from build123d import *

# Parameters (mm, degrees)
F1_DEPTH = 3
F2_DEPTH = 2.5
F3_R     = 4.5
F4_DEPTH = 1.25
F6_SIZE  = 1.24999
F5_R     = 1.75
F7_DEPTH = 1.35


# Not quite as in the source:
# - a fillet or chamfer is up to 0.001 mm smaller than in the source, because OpenCascade refuses the exact size


with BuildPart() as f1:
    # F0 (on Top) → F1 (new body)
    with BuildSketch(Plane.XY):
        with BuildLine():
            ThreePointArc((7.8345588235, -1.6185450382), (6.75, 0), (7.8345588235, 1.6185450382))
            ThreePointArc((7.8345588235, 1.6185450382), (7.7274066103, 2.0705523608), (7.5941994877, 2.5155782915))
            ThreePointArc((7.5941994877, 2.5155782915), (5.8456714755, 3.375), (5.9756544495, 5.318980532))
            ThreePointArc((5.9756544495, 5.318980532), (5.6568542495, 5.6568542495), (5.318980532, 5.9756544495))
            ThreePointArc((5.318980532, 5.9756544495), (3.375, 5.8456714755), (2.5155782915, 7.5941994877))
            ThreePointArc((2.5155782915, 7.5941994877), (2.0705523608, 7.7274066103), (1.6185450382, 7.8345588235))
            ThreePointArc((1.6185450382, 7.8345588235), (0, 6.75), (-1.6185450382, 7.8345588235))
            ThreePointArc((-1.6185450382, 7.8345588235), (-2.0705523608, 7.7274066103), (-2.5155782915, 7.5941994877))
            ThreePointArc((-2.5155782915, 7.5941994877), (-2.5038989162, 7.4779678276), (-2.5, 7.3612159322))
            ThreePointArc((-2.5, 7.3612159322), (-3.4780595655, 5.7906720883), (-5.318980532, 5.9756544495))
            ThreePointArc((-5.318980532, 5.9756544495), (-5.6568542495, 5.6568542495), (-5.9756544495, 5.318980532))
            ThreePointArc((-5.9756544495, 5.318980532), (-5.7048294141, 4.8146978862), (-5.6112159322, 4.25))
            ThreePointArc((-5.6112159322, 4.25), (-6.2090920721, 2.932764026), (-7.5941994877, 2.5155782915))
            ThreePointArc((-7.5941994877, 2.5155782915), (-7.7274066103, 2.0705523608), (-7.8345588235, 1.6185450382))
            ThreePointArc((-7.8345588235, 1.6185450382), (-7.0462080515, 0.9741606493), (-6.75, 0))
            ThreePointArc((-6.75, 0), (-7.0462080515, -0.9741606493), (-7.8345588235, -1.6185450382))
            ThreePointArc((-7.8345588235, -1.6185450382), (-7.7274066103, -2.0705523608), (-7.5941994877, -2.5155782915))
            ThreePointArc((-7.5941994877, -2.5155782915), (-6.2090920721, -2.932764026), (-5.6112159322, -4.25))
            ThreePointArc((-5.6112159322, -4.25), (-5.7048294141, -4.8146978862), (-5.9756544495, -5.318980532))
            ThreePointArc((-5.9756544495, -5.318980532), (-5.6568542495, -5.6568542495), (-5.318980532, -5.9756544495))
            ThreePointArc((-5.318980532, -5.9756544495), (-3.4780595655, -5.7906720883), (-2.5, -7.3612159322))
            ThreePointArc((-2.5, -7.3612159322), (-2.5038989162, -7.4779678276), (-2.5155782915, -7.5941994877))
            ThreePointArc((-2.5155782915, -7.5941994877), (-2.0705523608, -7.7274066103), (-1.6185450382, -7.8345588235))
            ThreePointArc((-1.6185450382, -7.8345588235), (0, -6.75), (1.6185450382, -7.8345588235))
            ThreePointArc((1.6185450382, -7.8345588235), (2.0705523608, -7.7274066103), (2.5155782915, -7.5941994877))
            ThreePointArc((2.5155782915, -7.5941994877), (3.375, -5.8456714755), (5.318980532, -5.9756544495))
            ThreePointArc((5.318980532, -5.9756544495), (5.6568542495, -5.6568542495), (5.9756544495, -5.318980532))
            ThreePointArc((5.9756544495, -5.318980532), (5.8456714755, -3.375), (7.5941994877, -2.5155782915))
            ThreePointArc((7.5941994877, -2.5155782915), (7.7274066103, -2.0705523608), (7.8345588235, -1.6185450382))
        make_face()
        Polygon((3.4641016151, 0), (1.7320508076, -3), (-1.7320508076, -3), (-3.4641016151, 0), (-1.7320508076, 3), (1.7320508076, 3), align=None, mode=Mode.SUBTRACT)
        Polygon((-1.7320508076, -3), (1.7320508076, -3), (3.4641016151, 0), (1.7320508076, 3), (-1.7320508076, 3), (-3.4641016151, 0), align=None)
    extrude(amount=F1_DEPTH)

    # F0 (on Top) → F2 (cut)
    with BuildSketch(Plane.XY):
        Polygon((-1.7320508076, -3), (1.7320508076, -3), (3.4641016151, 0), (1.7320508076, 3), (-1.7320508076, 3), (-3.4641016151, 0), align=None)
    extrude(amount=F2_DEPTH, mode=Mode.SUBTRACT)

    # F3 (on face) → F4 (join)
    with BuildSketch(Plane.XY.offset(3)):
        Circle(F3_R)
    extrude(amount=F4_DEPTH)

    # F6 (size 1.25 in the source; OpenCascade refuses exactly that, so slightly less here)
    f6_edges = [f1.edges().sort_by_distance(p)[0] for p in [
        (-4.5, 0, 4.25),
    ]]
    chamfer(f6_edges, length=F6_SIZE)

    # F5 (on face) → F7 (cut)
    with BuildSketch(Plane.XY.offset(4.25)):
        Circle(F5_R)
    extrude(amount=-F7_DEPTH, mode=Mode.SUBTRACT)


solid = f1.part
Input: part model. Units: mm. Frame: model coordinates. A direction names the side the tool comes from. Round coordinates to 2 decimals unless told otherwise and drop trailing zeros. Write each loop counter-clockwise with the first axis right and the second up, starting at its lowest first coordinate (ties: lowest second). Pieces come first, ordered by that corner, then holes.
1) Reachability of faces 4 (the flat face through (0, 0, 2.9)), 5 (the cylindrical face through (-7.726, 2.077, 1.479)), 6 (the flat face through (-2.6, -1.5, 1.2)) from +Z, -Z, +X, -X, +Y, -Y: full face, straight path, thin tool, end or side. Return the list, or none.
2) Draft query along Y for faces 1 (the cylindrical face through (2.06, -7.73, 1.48)), 2 (the cylindrical face through (1.617, -0.67, 3.584)), 3 (the flat face through (-4, 0, 0)). Return one class per face: pulls with the +Y half, pulls with the -Y half, needs draft (parallel to the pull), parting line crosses it, or undercut.
3) Cut plane B-B (z = 4.05). Return the cut outline in (x, y), then the cut area to 3 significant figures.
4) Contact query for flat-ended pins moving along their axis: P1, Ø1, axis at x = 0.5, y = 0, coming from the +Z side; P2, Ø3, axis at x = 0, y = 0, coming from the -Z side; P3, Ø1.2, axis at x = -0.5, z = 1, coming from the -Y side. Output: stop coordinate, or through.
5) Cut plane C-C (y = 6.25). Return the cut outline in (x, z), then the cut area to 3 significant figures.
6) Ray query, L1, parallel to Z at x = -2, y = 0.25; L2, parallel to Z at x = -7, y = -1; L3, parallel to Y at x = 0, z = 3.95. Return the intervals inside material, ascending.
Geometry says:
1. face 4: +Z
1. face 5: +Z, -Z, -X, +Y
1. face 6: -Z
2. face 1: pulls with the -Y half
2. face 2: undercut
2. face 3: needs draft
3. outline: circle Ø6.9 at (0, 0); hole circle Ø3.5 at (0, 0)
3. area: 27.8 mm2
4. P1: stops at z = 2.9
4. P2: stops at z = 2.5
4. P3: stops at y = -7.14
5. outline: (-2.9, 0) - (2.9, 0) - (2.9, 3) - (-2.9, 3) - close
5. area: 17.4 mm2
6. L1: z = 2.5 to 4.25
6. L2: z = 0 to 3
6. L3: y = -3.55 to -1.75, 1.75 to 3.55
